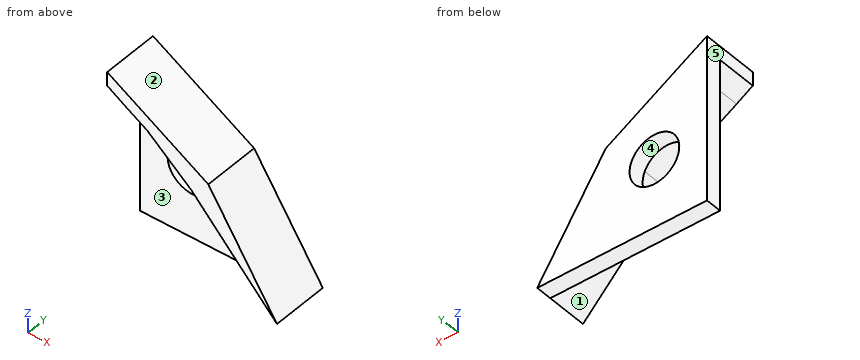
from build123d import *

# Parameters (mm, degrees)
SKETCH1_R           = 3.075
BOSS_EXTRUDE1_DEPTH = 2
BOSS_EXTRUDE2_DEPTH = 5


with BuildPart() as part:
    # Sketch1 → Boss-Extrude1 (new body)
    with BuildSketch(Plane(origin=(0, 0, 0), x_dir=(1, 0, 0), z_dir=(0, 1, 0))):
        Polygon((69.882295615, -141.15690287), (82.382295615, -133.65690287), (90.871460172, -120.65690287), (69.882295615, -120.65690287), align=None)
        with Locations(Location((76.382295615, -129.15690287, 0), (0, 0, 270))):
            Circle(SKETCH1_R, mode=Mode.SUBTRACT)
    extrude(amount=BOSS_EXTRUDE1_DEPTH)

    # Sketch2 → Boss-Extrude2 (add)
    with BuildSketch(Plane(origin=(0, 0, 0), x_dir=(-1, 0, 0), z_dir=(0, -1, 0))):
        Polygon((-69.882295615, -141.15690287), (-82.382295615, -133.65690287), (-90.871460172, -120.65690287), (-80.30000632, -131.836011395), (-74.842574052, -136.43145024), (-71.882295615, -138.207617302), (-69.882295615, -139.45690287), align=None)
    extrude(amount=BOSS_EXTRUDE2_DEPTH)


solid = part.part
Geometry check sheet. Reference: the model listing, model coordinates, mm. Face numbers are marked on the shaded views. A direction names the side the tool comes from. Give positions to 0.01 mm unless a question says otherwise; leave off trailing zeros. Write each loop counter-clockwise with the first axis right and the second up, starting at its lowest first coordinate (ties: lowest second). Pieces come first, ordered by that corner, then holes. Notation, with made-up numbers: M 1.25,16.5 L 8.25,16.5 A23 ccw 8.25,33.5 Z; hole C 45,-24 d2. An arc over 180 degrees is marked long. Answer as CSV lines item,"result". Start each with the question number.
Q1. Section check C-C, the plane x = 76.75. Record the cut outline in (y, z).
Q2. Release check for a two-part mould opening along X. For the marked faces 3, 4 and 5 record: pulls with the +X half, pulls with the -X half, needs draft (parallel to the pull), parting line crosses it, or undercut.
Q3. Section check A-A, the plane z = 128.5. Record the cut outline in (x, y), then the cut area to 3 significant figures.
Q4. Go/stop test with flat-tipped pins: pin 1 (1 mm diameter, centred on x = 78.5, z = 126, fed in from -Y); pin 2 (1 mm diameter, centred on x = 84, y = -3, fed in from -Z); pin 3 (4 mm diameter, centred on x = 72.5, y = -2, fed in from +Z). Record where each tip stops, or that it passes through.
Q5. Section check D-D, the plane y = 1. Record the cut outline in (x, z) (3 decimals), then the cut area to 3 significant figures.
Q6. Material ranges on L1, parallel to Y at x = 86.5, z = 123.25; L2, parallel to Z at x = 75, y = 0.5; L3, parallel to Z at x = 77, y = 0.25, recorded low to high.
Q7. Tool access check on the marked faces 1 and 2. Record the directions out of +Z, -Z, +X, -X, +Y, -Y that give a thin tool (end or side, any length) a straight path to the whole face; none if there is none.
Q8. Section check B-B, the plane y = -3. Record the cut outline in (x, z), then the cut area to 3 significant figures.
Geometry says:
1,outline,"M -5,134.83 L 0,134.83 L 0,132.21 L 2,132.21 L 2,137.04 L -5,137.04 Z; M 0,120.66 L 2,120.66 L 2,126.1 L 0,126.1 Z"
2,face 3,"needs draft"
2,face 4,"undercut"
2,face 5,"pulls with the -X half"
3,outline,"M 69.88,0 L 73.38,0 L 73.38,2 L 69.88,2 Z; M 79.39,0 L 83.45,0 L 83.45,-5 L 85.75,-5 L 85.75,2 L 79.39,2 Z"
3,area,"31.2 mm^2"
4,pin 1,"y = 0"
4,pin 2,"z = 127.39"
4,pin 3,"z = 140.79"
5,outline,"M 69.882,120.657 L 90.871,120.657 L 82.382,133.657 L 69.882,141.157 Z; hole C 76.382,129.157 d6.15"
5,area,"235 mm^2"
6,L1,"0 to 2"
6,L2,"120.66 to 126.41, 131.9 to 138.09"
6,L3,"120.66 to 126.14, 132.17 to 136.89"
7,face 1,"-Z, -X, -Y"
7,face 2,"+Z, +X, +Y, -Y"
8,outline,"M 69.88,139.46 L 71.88,138.21 L 74.84,136.43 L 80.3,131.84 L 90.87,120.66 L 82.38,133.66 L 69.88,141.16 Z"
8,area,"46.2 mm^2"
